Source: CAD feature listing. Evaluate the final solid. Frame: model axes, mm. A direction names the side the tool comes from. Round coordinates to 2 decimals unless told otherwise and drop trailing zeros. Order: outer loops, then holes, each group sorted by start corner. A loop starts at its lowest first (then second) coordinate and runs counter-clockwise, first axis right, second up. Notation, with made-up numbers: (18.25, -17) -> (22.25, -17) arc R20 cw to (22.25, 3) -> close; hole circle Ø7 at (3.5, 31). An arc over 180 degrees is marked (long way). Write item = value, one per line. Start each with the question number.
(1) Draft query along X for faces 1 (the face through (-2.744, -7, 7)), 2 (the face through (7.375, -11.976, 2.549)), 3 (the face through (16.516, -10.978, 13.496)). Return one class per face: released by +X, released by -X, zero draft, split by the parting line, or undercut.
(2) Cut plane B-B on x = 7. Return the cut outline in (y, z), then the cut area to 3 significant figures.
(3) Ray query, line 1 (X direction, y = -9.25, z = 4.5); line 2 (Z direction, x = 8.75, y = -6.5); line 3 (X direction, y = -4, z = 12.5). Return the intervals inside material, ascending.
(4) Cut plane C-C on z = 9. Return the cut outline in (x, y), then the cut area to 3 significant figures.
(5) Reachability of faces 4 (the face through (14.68, -11.95, 6.63)), 5 (the face through (17.256, -7, 7)), 6 (the face through (7, -12.404, 1)), 7 (the face through (14.256, -7, 8)), 8 (the face through (-0.195, -2.832, 5.81)) from +Z, -Z, +X, -X, +Y, -Y: full face, straight path, thin tool, end or side. Return the list, or none.
(6) Cut plane A-A on z = 6.75. Return the cut outline in (x, y).
(7) Contact query for flat-ended pins moving along their axis: pin 1 Ø8 at (x, z) = (0.5, 9) entering from -Y; pin 2 Ø3.5 at (x, y) = (5, -7) entering from +Z. Output: stop coordinate, or through.
from build123d import *

# Parameters (mm, degrees)
F1_DEPTH = 3
F2_W     = 3
F2_H     = 10
F3_DEPTH = 12
F5_DEPTH = 25
F6_R     = 4.99999
F7_R     = 1.5


# Not quite as in the source:
# - a fillet or chamfer is up to 0.001 mm smaller than in the source, because OpenCascade refuses the exact size


with BuildPart() as f1:
    # F0 (on Top) → F1 (new body)
    with BuildSketch(Plane.XY):
        with BuildLine():
            Line((5.7057162493, -7.4039038014), (-2.7442837507, -7.4039038014))
            Line((-2.7442837507, -7.4039038014), (-2.7442837507, -12.4039038014))
            Line((-2.7442837507, -12.4039038014), (7.2557162493, -12.4039038014))
            Line((7.2557162493, -12.4039038014), (7.2557162493, -8.9539038014))
            ThreePointArc((7.2557162493, -8.9539038014), (6.1597007385, -8.4999193123), (5.7057162493, -7.4039038014))
        make_face()
        with BuildLine():
            Line((17.2557162493, -2.4039038014), (-2.7442837507, -2.4039038014))
            Line((-2.7442837507, -2.4039038014), (-2.7442837507, -7.4039038014))
            Line((-2.7442837507, -7.4039038014), (5.7057162493, -7.4039038014))
            ThreePointArc((5.7057162493, -7.4039038014), (7.2557162493, -5.8539038014), (8.8057162493, -7.4039038014))
            ThreePointArc((8.8057162493, -7.4039038014), (8.3517317602, -8.4999193123), (7.2557162493, -8.9539038014))
            Line((7.2557162493, -8.9539038014), (7.2557162493, -12.4039038014))
            Line((7.2557162493, -12.4039038014), (17.2557162493, -12.4039038014))
            Line((17.2557162493, -12.4039038014), (17.2557162493, -2.4039038014))
        make_face()
    extrude(amount=F1_DEPTH)

    # F2 (on face) → F3 (join)
    with BuildSketch(Plane.XY.offset(3)):
        with Locations((-1.2442837507, -7.4039038014)):
            Rectangle(F2_W, F2_H)
        with Locations((15.7557162493, -7.4039038014)):
            Rectangle(F2_W, F2_H)
    extrude(amount=F3_DEPTH)

    # F4 (on face) → F5 (cut)
    with BuildSketch(Plane(origin=(-2.7442837507, 0, 0), x_dir=(0, -1, 0), z_dir=(-1, 0, 0))):
        with BuildLine():
            ThreePointArc((5.8539038014, 10), (6.3078882906, 8.9039844892), (7.4039038014, 8.45))
            Line((7.4039038014, 8.45), (7.4039038014, 10))
            Line((7.4039038014, 10), (5.8539038014, 10))
        make_face()
        with BuildLine():
            Line((7.4039038014, 10), (7.4039038014, 8.45))
            ThreePointArc((7.4039038014, 8.45), (8.4999193123, 8.9039844892), (8.9539038014, 10))
            ThreePointArc((8.9539038014, 10), (7.4039038014, 11.55), (5.8539038014, 10))
            Line((5.8539038014, 10), (7.4039038014, 10))
        make_face()
    extrude(amount=-F5_DEPTH, mode=Mode.SUBTRACT)

    # F6 (radius 5 in the source; OpenCascade refuses exactly that, so slightly less here)
    f6_edges = [f1.edges().sort_by_distance(p)[0] for p in [
        (-1.244284, -2.403904, 15),
        (15.755716, -2.403904, 15),
        (15.755716, -12.403904, 15),
        (-1.244284, -12.403904, 15),
    ]]
    fillet(f6_edges, radius=F6_R)

    # F7
    f7_edges = [f1.edges().sort_by_distance(p)[0] for p in [
        (7.255716, -2.403904, 3),
        (7.255716, -12.403904, 3),
        (0.255716, -10.939441, 13.535537),
        (14.255716, -3.868367, 13.535537),
    ]]
    fillet(f7_edges, radius=F7_R)


solid = f1.part
Evaluation:
q1.face_1 = released by -X
q1.face_2 = undercut
q1.face_3 = zero draft
q2.outline = (-12.4, 0) -> (-8.93, 0) -> (-8.93, 3) -> (-10.9, 3) arc R1.5 ccw to (-12.4, 1.5) -> close; (-5.88, 0) -> (-2.4, 0) -> (-2.4, 1.5) arc R1.5 ccw to (-3.9, 3) -> (-5.88, 3) -> close
q2.area = 19.9 mm^2
q3.line_1 = -2.74 to 0.26, 14.26 to 17.26
q3.line_2 = 0 to 3
q3.line_3 = -2.74 to 0.07, 14.44 to 17.26
q4.outline = (-2.74, -12.4) -> (-1.24, -12.4) arc R1.5 ccw to (0.26, -10.9) -> (0.26, -8.59) -> (-2.74, -8.59) -> close; (-2.74, -6.22) -> (0.26, -6.22) -> (0.26, -3.9) arc R1.5 ccw to (-1.24, -2.4) -> (-2.74, -2.4) -> close; (14.26, -10.9) arc R1.5 ccw to (15.76, -12.4) -> (17.26, -12.4) -> (17.26, -8.59) -> (14.26, -8.59) -> close; (14.26, -6.22) -> (17.26, -6.22) -> (17.26, -2.4) -> (15.76, -2.4) arc R1.5 ccw to (14.26, -3.9) -> close
q4.area = 43.9 mm^2
q5.face_4 = +Z, -Y
q5.face_5 = +Z, -Z, +X, +Y, -Y
q5.face_6 = +Z, -Z, +X, -X, -Y
q5.face_7 = +Z, +Y, -Y
q5.face_8 = +Z, +Y
q6.outline = (-2.74, -12.4) -> (-1.24, -12.4) arc R1.5 ccw to (0.26, -10.9) -> (0.26, -3.9) arc R1.5 ccw to (-1.24, -2.4) -> (-2.74, -2.4) -> close; (14.26, -10.9) arc R1.5 ccw to (15.76, -12.4) -> (17.26, -12.4) -> (17.26, -2.4) -> (15.76, -2.4) arc R1.5 ccw to (14.26, -3.9) -> close
q7.pin_1 = -12.4
q7.pin_2 = 3
